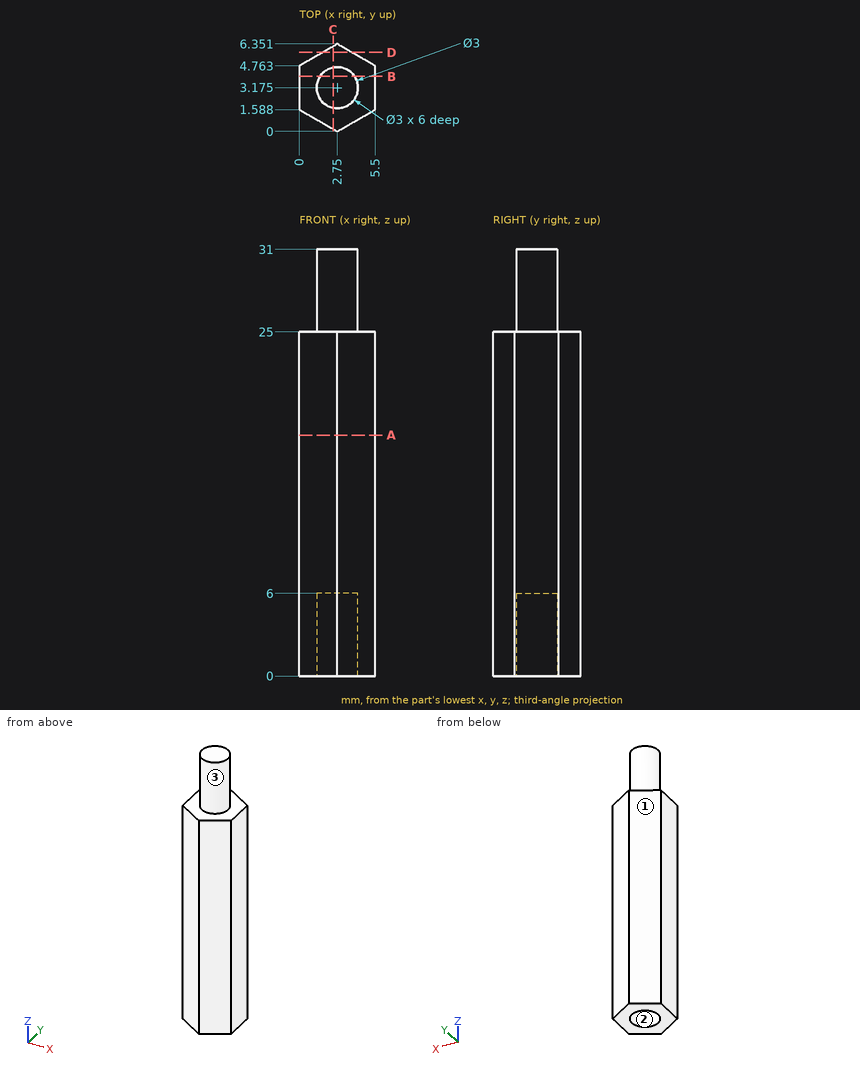
Geometry check sheet. Reference: drawing and pictorial views, mm from the part's lowest x, y, z. Give positions to 0.01 mm unless a question says otherwise; leave off trailing zeros. Loops run counter-clockwise (first coordinate to the right, second up) from the corner with the lowest first, then second, coordinate; pieces in that order, holes last.
1. Section check A-A, the plane z = 17.5. Enter the section's corners in (x, y), then the cut area to 3 significant figures.
2. Section check D-D, the plane y = 5.75. Enter the section's corners in (x, z).
3. Mould release check, pull along X, two halves, no side actions. Record for the marked faces 1, 2 and 3: released by +X, released by -X, zero draft, split by the parting line, or undercut.
4. Section check C-C, the plane x = 2.45. Enter the section's corners in (y, z) (1 decimal), then the cut area to 3 significant figures.
5. Thickness scan on line 1 (Z direction, x = 4.6, y = 1.5); line 2 (Y direction, x = 2.2, z = 4) (1 decimal); line 3 (Y direction, x = 0.8, z = 16) (1 decimal). Record the ranges inside material, lowest first.
6. Go/stop test with a flat-tipped pin: pin 1 Ø2.5 at (x, y) = (2.75, 3.18) entering from -Z. Record where the tip stops, or that it passes through.
7. Section check B-B, the plane y = 4. Enter the section's corners in (x, z).
Geometry says:
1. outline: (0, 1.59) - (2.75, 0) - (5.5, 1.59) - (5.5, 4.76) - (2.75, 6.35) - (0, 4.76) - close
1. area: 26.2 mm2
2. outline: (1.71, 0) - (3.79, 0) - (3.79, 25) - (1.71, 25) - close
3. face 1: released by -X
3. face 2: undercut
3. face 3: split by the parting line
4. outline: (0.2, 0) - (1.7, 0) - (1.7, 6) - (4.6, 6) - (4.6, 0) - (6.2, 0) - (6.2, 25) - (4.6, 25) - (4.6, 31) - (1.7, 31) - (1.7, 25) - (0.2, 25) - close
4. area: 150 mm2
5. line 1: z = 0 to 25
5. line 2: y = 0.3 to 1.8, 4.6 to 6
5. line 3: y = 1.1 to 5.2
6. pin 1: stops at z = 6
7. outline: (0, 0) - (1.5, 0) - (1.5, 6) - (4, 6) - (4, 0) - (5.5, 0) - (5.5, 25) - (4, 25) - (4, 31) - (1.5, 31) - (1.5, 25) - (0, 25) - close
